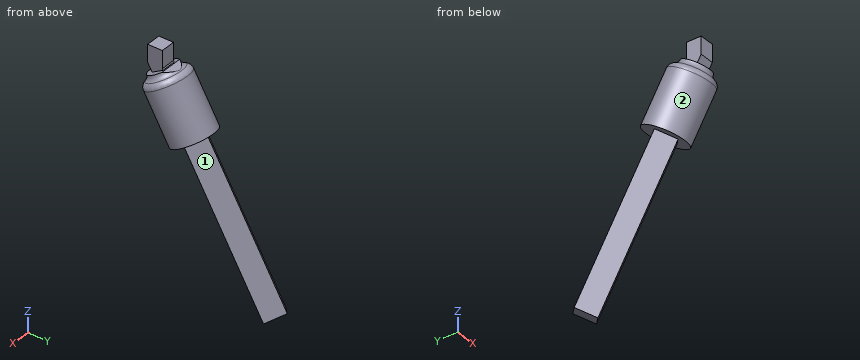
Autodesk Inventor part; units mm, degrees
ref_plane "Plan de construction1" through (0, 0, 5) normal (0, -0.5, 0.8660254) x (1, 0, 0)
ref_plane "Plan de construction2" through (5, 5, 0) normal (0, 0.5, -0.8660254) x (-1, 0, 0)
ref_plane "YZ Plane" through (0, 0, 0) normal (1, 0, 0) x (0, 1, 0)
sketch "Esquisse1" plane through (0, 0, 0) normal (0, 0, 1) x (1, 0, 0)
  line L0 (0, 0) -> (5, 0)
  line L1 (5, 0) -> (5, 5)
  line L2 (5, 5) -> (0, 5)
  line L3 (0, 5) -> (0, 0)
  dimension "d0" = 5
  dimension "d1" = 5
extrude "Extrusion1" add sketch "Esquisse1" along normal blind 5
ref_plane "Plan de construction1" through (0, 0, 5) normal (0, -0.5, 0.8660254) x (1, 0, 0)
sketch "Esquisse2" plane through (0, 0, 5) normal (0, -0.5, 0.8660254) x (1, 0, 0)
  line L0 (0, 4.3301) -> (5, 4.3301)
  line L1 (5, 0) -> (5, 4.3301)
  line L2 (0, 4.3301) -> (5, 4.3301)
  line L3 (5, 4.3301) -> (5, 0)
  line L4 (5, 0) -> (0, 0)
  line L5 (0, 0) -> (0, 4.3301)
  point P0 (0, -2.5)
extrude "Extrusion2" add sketch "Esquisse2" along normal mid plane 5
sketch "Esquisse3" plane through (0, -1.25, 7.1651) normal (0, -0.5, 0.8660254) x (1, 0, 0)
  line L0 (0, 0) -> (5, 0)
  line L1 (5, 0) -> (5, 4.3301)
  line L2 (5, 4.3301) -> (0, 4.3301)
  line L3 (0, 4.3301) -> (0, 0)
  point P0 (0, -2.5)
extrude "Extrusion3" add sketch "Esquisse3" along normal blind 5
fillet "Congé1" radius 2 2 edges at (2.5, 0, 13.6603) (2.5, -3.75, 11.4952)
ref_plane "Plan de construction2" through (5, 5, 0) normal (0, 0.5, -0.8660254) x (-1, 0, 0)
sketch "Esquisse4" plane through (5, 5, 0) normal (0, 0.5, -0.8660254) x (-1, 0, 0)
  line L0 (0, 0) -> (0, 2.5)
  line L1 (5, -4.3301) -> (5, -1.8301)
  line L2 (0, 0) -> (5, 0)
  line L3 (5, 0) -> (5, -4.3301)
  line L4 (5, -4.3301) -> (0, -4.3301)
  line L5 (0, -4.3301) -> (0, 0)
  point P0 (5, -1.8301)
extrude "Extrusion4" add sketch "Esquisse4" along normal mid plane 5
sketch "Esquisse6" plane through (5, 6.25, -2.1651) normal (0, 0.5, -0.8660254) x (-1, 0, 0)
  line L0 (0, 0) -> (5, 0)
  line L1 (5, 0) -> (2.5, 0)
  line L2 (2.5, 0) -> (2.5, -2.165)
  circle A0 centre (2.5, -2.165) radius 5
  point P0 (5, -4.3301)
  dimension "d14" = 2.165
  dimension "d15" = 10
extrude "Extrusion5" add sketch "Esquisse6" against normal blind 2
sketch "Esquisse7" plane through (5, 5, 5) normal (1, 0, 0) x (0, 0, -1)
  line L0 (5.433, 0.25) -> (5, 0)
  line L1 (5, 0) -> (-0.081, 0)
  line L2 (-0.081, 0) -> (-0.081, 15.1439)
  line L3 (-0.081, 15.1439) -> (5, 15.1439)
  line L4 (5, 15.1439) -> (5, 0)
  point P0 (5, -5)
extrude "Extrusion6" cut sketch "Esquisse7" along normal through all both and the other way through all
sketch "Esquisse8" plane through (2.5, 4.3751, -3.2476) normal (0, 0.5, -0.8660254) x (-1, 0, 0)
  arc A0 (3.9765, 3.031) -> (-3.9765, 3.031) centre (0, 0) ccw
  line L0 (0, 5) -> (-5, 0)
  arc A1 (-3.9765, 3.031) -> (3.9765, 3.031) centre (0, 0) ccw
  line L1 (0, -5) -> (-5, 0)
  line L2 (0, -5) -> (5, 0)
  line L3 (5, 0) -> (0, 5)
  point P0 (2.5, -2.1651)
extrude "Extrusion7" add sketch "Esquisse8" along normal blind 74.5 contours L3 L2 L1 L0
sketch "Esquisse9" plane through (5, 6.25, -2.1651) normal (0, 0.5, -0.8660254) x (-1, 0, 0)
  line L0 (7.5, -2.165) -> (2.5, 2.835)
  arc A0 (-1.4765, 0.866) -> (6.4765, 0.866) centre (2.5, -2.165) ccw
  arc A1 (6.4765, 0.866) -> (-1.4765, 0.866) centre (2.5, -2.165) ccw
  circle A2 centre (2.5, -2.165) radius 7.5
  point P0 (5, -4.3301)
  dimension "d24" = 15
extrude "Extrusion8" add sketch "Esquisse9" along normal blind 19.5 contours A0 A1 L0 | L0 A1 A0 | A2
fillet "Congé2" radius 2 1 edges at (7.5, 4.3751, -3.2476)
fillet "Congé3" radius 2 1 edges at (10, 4.3751, -3.2476)
sketch "Esquisse10" plane through (5, 5, 5) normal (1, 0, 0) x (0, 0, -1)
  line L0 (0, 0) -> (-6.9282, -4)
  line L1 (0, 0) -> (-8.5321, 0)
  line L2 (-8.5321, 0) -> (-8.5321, -9.6747)
  line L3 (-8.5321, -9.6747) -> (0, -9.6747)
  line L4 (0, -9.6747) -> (0, 0)
  point P0 (5, -5)
extrude "Extrusion9" cut sketch "Esquisse10" against normal through all
sketch "Esquisse11" plane through (5, 0, 5) normal (0, 0, 1) x (1, 0, 0)
  line L0 (-5, 0) -> (0, 0)
  line L1 (0, 5) -> (0, 0)
  line L2 (0, 5) -> (-5, 5)
  line L3 (-5, 0) -> (-5, 5)
  line L4 (-5, 0) -> (0, 0)
  line L5 (0, 5) -> (0, 0)
  line L6 (0, 5) -> (-5, 5)
  line L7 (-5, 0) -> (-5, 5)
extrude "Extrusion10" add sketch "Esquisse11" along normal blind 1
properties part number "Bras hélice"
Geometry: final body of the model. Coordinates: model frame, mm. Face numbers are marked on the shaded views. A direction names the side the tool comes from. Round coordinates to 2 decimals unless told otherwise and drop trailing zeros. Loops run counter-clockwise (first coordinate to the right, second up) from the corner with the lowest first, then second, coordinate; pieces in that order, holes last. Notation, with made-up numbers: M -31,-33 L -10,-33 A35 cw -10,2 Z; hole C -11,-17 d8. An arc over 180 degrees is marked long. Put each result on its own line as item: value. Start each with the question number.
(1) Section query A-A (y = 39.5). Return loops of the section in (x, z), then the cut area to 3 significant figures.
(2) Contact query for flat-ended pins moving along their axis: pin 1 Ø6 at (y, z) = (21, -31.5) entering from -X; pin 2 Ø5 at (x, z) = (1, -12.5) entering from -Y; pin 3 Ø3.5 at (x, y) = (2, 7) entering from +Z. Output: stop coordinate, or through.
(3) Section query B-B (z = -48). Return loops of the section in (x, y), then the cut area to 3 significant figures.
(4) Material intervals for line 1 along Y through (x, z) = (-0.25, -22.5); line 2 along Z through (x, y) = (1, 17.5); line 3 along Z through (x, y) = (0.25, 20.5), sorted ascending. Write a range as [from, to].
(5) Section query C-C (y = 29.5). Return loops of the section in (x, z), then the cut area to 3 significant figures.
(6) Set-up query: the marked faces 1 and 2. Return all of +Z, -Z, +X, -X, +Y, -Y with unobstructed straight access to the full face (end or side cutting, diameter ignored); none if empty.
Findings below:
1. outline: M -2.5,-64.09 L -0.05,-68.99 L 5.05,-68.99 L 7.5,-64.09 L 2.5,-54.09 Z
1. area: 87.0 mm2
2. pin 1: stops at x = -2.5
2. pin 2: stops at y = -0.28
2. pin 3: stops at z = 0
3. outline: M -2.5,30.21 L 2.5,24.44 L 7.5,30.21 L 2.5,35.99 Z
3. area: 57.7 mm2
4. line 1: y = [7.43, 10.03], [12.89, 18.09]
4. line 2: z = [-32.98, -18.98], [-18.19, -11.28]
4. line 3: z = [-36.68, -25.68]
5. outline: M -2.5,-46.77 L 2.5,-56.77 L 7.5,-46.77 L 2.5,-36.77 Z
5. area: 100 mm2
6. face 1: +X, +Y
6. face 2: none
